Here's how the part is built. I have some questions about the finished solid (model axes, mm). A direction names the side the tool comes from. Coordinates: 2 decimals unless noted, no trailing zeros. Write each loop counter-clockwise with the first axis right and the second up, starting at its lowest first coordinate (ties: lowest second). Pieces come first, ordered by that corner, then holes.
Item 1: I'm going to push flat-ended pins straight in: pin 1 Ø1 at (y, z) = (15, -12.5) entering from -X; pin 2 Ø2 at (y, z) = (41.5, -8) entering from +X; pin 3 Ø13 at (x, y) = (13, 22.5) entering from -Z. Where does each tip first touch, or does it pass through?
Item 2: If we section it at D-D (y = 54): Please give me the cut outline in (x, z).
Item 3: If we section it at B-B (x = 9): Please give me the cut outline in (y, z), then the cut area to 3 significant figures.
Item 4: We'd pull the mould along X, two halves only. Please class faces 4 (the face through (24.39, 51.94, -1.01)), 5 (the face through (2, 30, -12)), 6 (the face through (1, 54, -9)): +X half, -X half, draft (parallel to the pull), parting line (faces both ways), or undercut.
Item 5: For faces 1 (the face through (17, 30, -2)), 2 (the face through (1, 7, -15)), 3 (the face through (30, 30, -1)), which set-ups out of +Z, -Z, +X, -X, +Y, -Y let a thin tool reach every point of the face, with its end or its side?
Item 6: If we section it at C-C (y = 35): Please give me the cut outline in (x, z), then the cut area to 3 significant figures.
Item 7: If we section it at A-A (z = -10.75): Please give me the cut outline in (x, y), then the cut area to 3 significant figures.
Item 8: If I drill on line 1 (Y direction, x = 23, z = -0.4); line 2 (Y direction, x = 1.5, z = -16.5); line 3 (Z direction, x = 21.5, y = 48), over which ranges is the centre line in solid material (lowest first)?
from build123d import *

# Parameters (mm, degrees)
BOSS_EXTRU_1_DEPTH      = 60
ENL_V_MAT_EXTRU_1_DEPTH = 71
ESQUISSE3_R             = 1.75
ENL_V_MAT_EXTRU_2_DEPTH = 70.455021417
CONG_1_R                = 2


with BuildPart() as part:
    # Esquisse1 → Boss.-Extru.1 (new body)
    with BuildSketch(Plane(origin=(0, 0, 0), x_dir=(1, 0, 0), z_dir=(0, 1, 0))):
        Polygon((30, 0), (0, 0), (0, 20), (2, 20), (2, 2), (30, 2), align=None)
    extrude(amount=BOSS_EXTRU_1_DEPTH)

    # Esquisse2 → Enlèv. mat.-Extru.1 (cut, through all)
    with BuildSketch(Plane.ZY):
        with BuildLine():
            Line((-20, 55), (-10, 55))
            ThreePointArc((-10, 55), (-9, 54), (-10, 53))
            Line((-10, 53), (-20, 53))
            Line((-20, 53), (-20, 55))
        make_face()
        with BuildLine():
            Line((-20, 5), (-10, 5))
            ThreePointArc((-10, 5), (-9, 6), (-10, 7))
            Line((-10, 7), (-20, 7))
            Line((-20, 7), (-20, 5))
        make_face()
    extrude(amount=-ENL_V_MAT_EXTRU_1_DEPTH, mode=Mode.SUBTRACT)

    # Esquisse3 → Enlèv. mat.-Extru.2 (cut, through all)
    with BuildSketch(Plane(origin=(0, 0, -2), x_dir=(-1, 0, 0), z_dir=(0, 0, -1))):
        with Locations((-23, 53)):
            Circle(ESQUISSE3_R)
        with Locations((-9, 53)):
            Circle(ESQUISSE3_R)
        with Locations((-9, 7)):
            Circle(ESQUISSE3_R)
        with Locations((-23, 7)):
            Circle(ESQUISSE3_R)
    extrude(amount=-ENL_V_MAT_EXTRU_2_DEPTH, mode=Mode.SUBTRACT)

    # Congé1
    cong_1_edges = [part.edges().sort_by_distance(p)[0] for p in [
        (0, 30, 0),
        (2, 30, -2),
        (1, 60, -20),
        (30, 60, -1),
        (1, 0, -20),
        (30, 0, -1),
    ]]
    fillet(cong_1_edges, radius=CONG_1_R)


solid = part.part
Answer list:
1. pin 1: stops at x = 0
1. pin 2: stops at x = 2
1. pin 3: stops at z = -2
2. outline: (0, -9) - (2, -9) - (2, -4) arc R2 cw to (4, -2) - (7.56, -2) - (7.56, 0) - (2, 0) arc R2 ccw to (0, -2) - close; (10.44, -2) - (21.56, -2) - (21.56, 0) - (10.44, 0) - close; (24.44, -2) - (30, -2) - (30, 0) - (24.44, 0) - close
3. outline: (0, -2) - (5.25, -2) - (5.25, 0) - (0, 0) - close; (8.75, -2) - (51.25, -2) - (51.25, 0) - (8.75, 0) - close; (54.75, -2) - (60, -2) - (60, 0) - (54.75, 0) - close
3. area: 106 mm2
4. face 4: undercut
4. face 5: +X half
4. face 6: draft
5. face 1: -Z, +X, +Y, -Y
5. face 2: -Z, +X, -X
5. face 3: +Z, -Z, +X, +Y, -Y
6. outline: (0, -20) - (2, -20) - (2, -4) arc R2 cw to (4, -2) - (30, -2) - (30, 0) - (2, 0) arc R2 ccw to (0, -2) - close
6. area: 96.0 mm2
7. outline: (0, 0) - (2, 0) - (2, 5) - (0, 5) - close; (0, 7) - (2, 7) - (2, 53) - (0, 53) - close; (0, 55) - (2, 55) - (2, 60) - (0, 60) - close
7. area: 112 mm2
8. line 1: y = 0 to 5.25, 8.75 to 51.25, 54.75 to 60
8. line 2: y = 0 to 5, 7 to 53, 55 to 60
8. line 3: z = -2 to 0
